The drawing under review shows one solid part. Ordinate dimensions are in mm from its lowest x, y, z. Coordinates: 2 decimals unless noted, no trailing zeros. Write each loop counter-clockwise with the first axis right and the second up, starting at its lowest first coordinate (ties: lowest second). Pieces come first, ordered by that corner, then holes.
Q1. Take a section at C-C (z = 11). Give the boundary of the cut face in (x, y).
Q2. Take a section at A-A (x = 7). Give the boundary of the cut face in (y, z).
Q3. Insertion check: pin 1 (1 mm diameter, centred on x = 11.5, y = 5.5, fed in from -Z); pin 2 (1 mm diameter, centred on y = 5, z = 10, fed in from -X); pin 3 (2 mm diameter, centred on y = 3, z = 2, fed in from -X) (1 decimal). Each pin has a flat end and moves straight along its axis. Give the tip position at first contact, or say it passes through.
Q4. For probe 1 along Y at (x, z) = (7, 5.75); probe 2 along X at (y, z) = (3.75, 13); probe 3 along Y at (x, z) = (8.5, 11), list the stretches that pass through material, from the lowest coordinate up.
Q5. Mouldability with a two-part tool opening along X and no side actions: class the marked faces 1, 2 and 3 as pulls with the +X half, pulls with the -X half, needs draft (parallel to the pull), parting line crosses it, or undercut.
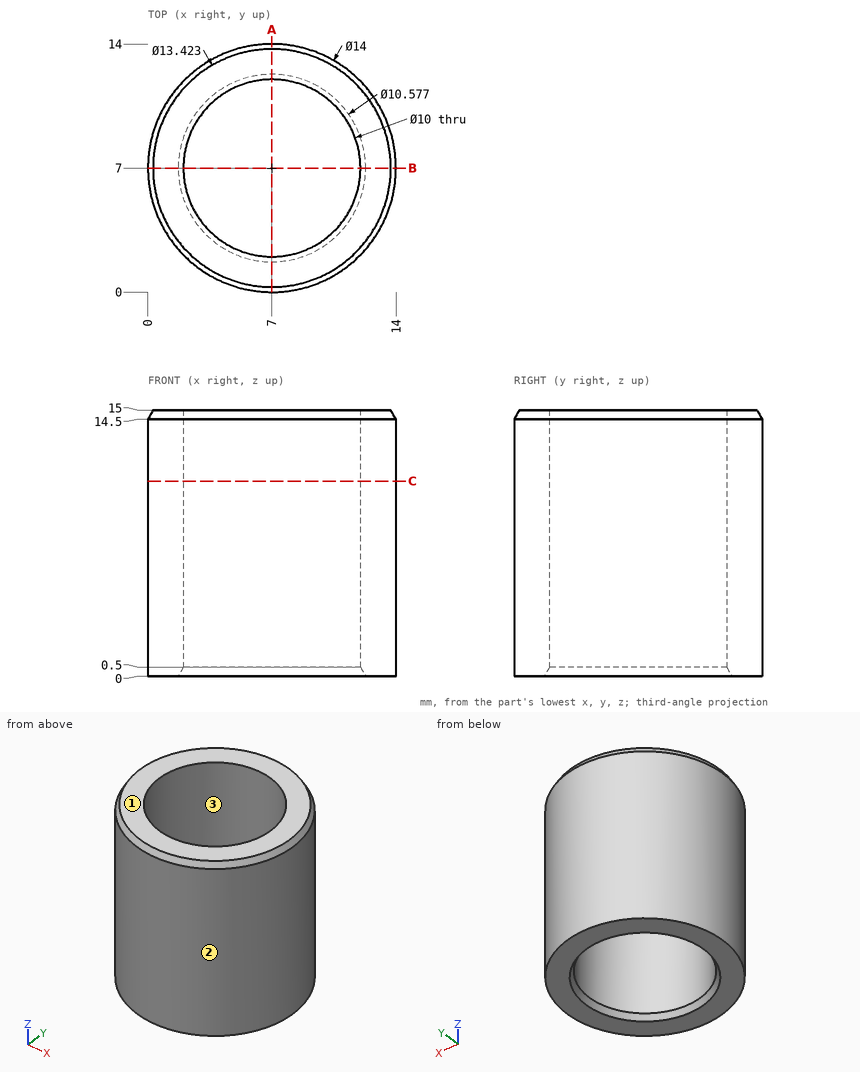
Response:
1. outline: circle Ø14 at (7, 7); hole circle Ø10 at (7, 7)
2. outline: (0, 0) - (1.71, 0) - (2, 0.5) - (2, 15) - (0.29, 15) - (0, 14.5) - close; (12, 0.5) - (12.29, 0) - (14, 0) - (14, 14.5) - (13.71, 15) - (12, 15) - close
3. pin 1: stops at z = 0.08
3. pin 2: stops at x = 0.16
3. pin 3: stops at x = 0.7
4. probe 1: y = 0 to 2, 12 to 14
4. probe 2: x = 0.8 to 3.2, 10.8 to 13.2
4. probe 3: y = 0.16 to 2.23, 11.77 to 13.84
5. face 1: needs draft
5. face 2: parting line crosses it
5. face 3: undercut
